Build history of the part. All positions in model axes, mm. A direction names the side the tool comes from. Round coordinates to 2 decimals unless told otherwise and drop trailing zeros. Order: outer loops, then holes, each group sorted by start corner. A loop starts at its lowest first (then second) coordinate and runs counter-clockwise, first axis right, second up. Notation, with made-up numbers: M 36.5,3 L 71.5,3 A14 ccw 71.5,7 Z; hole C -23.75,-25 d9. An arc over 180 degrees is marked long. Use CSV: the item, a comma, the result in double quotes.
from build123d import *

# Parameters (mm, degrees)
SKETCH1_R           = 2.95
SKETCH1_R_2         = 20
SKETCH1_R_3         = 18.5
BOSS_EXTRUDE1_DEPTH = 5.9
CUT_EXTRUDE2_DEPTH  = 78.081470808


with BuildPart() as part:
    # Sketch1 → Boss-Extrude1 (new body)
    with BuildSketch(Plane.XY):
        Polygon((-32.5, 4.1), (-32.5, -22), (32.5, -22), (32.5, 4.1), (54.344931419, 4.1), (54.344931419, 54.344931419), (-54.344931419, 54.344931419), (-54.344931419, 4.1), align=None)
        Circle(SKETCH1_R, mode=Mode.SUBTRACT)
        with Locations((29.344931419, 29.344931419)):
            Circle(SKETCH1_R_2, mode=Mode.SUBTRACT)
        with Locations((-29.344931419, 29.344931419)):
            Circle(SKETCH1_R_3, mode=Mode.SUBTRACT)
    extrude(amount=BOSS_EXTRUDE1_DEPTH)

    # Sketch3 → Cut-Extrude2 (cut, through all)
    with BuildSketch(Plane.XY.offset(5.9)):
        Polygon((-12.15, -22), (-7.85, -22), (-7.85, -17), (-5.4, -17), (-5.4, -14), (-7.85, -14), (-7.85, -10), (-12.15, -10), (-12.15, -14), (-14.6, -14), (-14.6, -17), (-12.15, -17), align=None)
        Polygon((7.85, -14), (7.85, -10), (12.15, -10), (12.15, -14), (14.6, -14), (14.6, -17), (12.15, -17), (12.15, -22), (7.85, -22), (7.85, -17), (5.4, -17), (5.4, -14), align=None)
    extrude(amount=-CUT_EXTRUDE2_DEPTH, mode=Mode.SUBTRACT)


solid = part.part
(1) Two-plate mould, pull along X, no slides. Class faces 1 (the face through (1, 54.345, 3)), 2 (the face through (-32.5, -9, 3)), 3 (the face through (32.5, -9, 3)), 4 (the face through (-14.6, -15, 3)): released by +X, released by -X, zero draft, split by the parting line, or undercut.
Answer block:
face 1,"zero draft"
face 2,"released by -X"
face 3,"released by +X"
face 4,"undercut"
(2) Cut at D-D, the plane y = 28. Give the cut face in (x, z).
Answer block:
outline,"M -54.34,0 L -47.8,0 L -47.8,5.9 L -54.34,5.9 Z; M -10.89,0 L 9.39,0 L 9.39,5.9 L -10.89,5.9 Z; M 49.3,0 L 54.34,0 L 54.34,5.9 L 49.3,5.9 Z"
(3) Wall check: line 1 (Y direction, x = 0, z = 3.55); line 2 (Y direction, x = 13, z = 5.2); line 3 (Y direction, x = -13, z = 1.35). Give the ranges that are in metal, low to high. Write a range as from..to.
Answer block:
line 1,"y = -22..-2.95, 2.95..54.34"
line 2,"y = -22..-17, -14..17.82, 40.87..54.34"
line 3,"y = -22..-17, -14..20.68, 38.01..54.34"
(4) Cut at C-C, the plane y = 12. Give the cut face in (x, z), and give its area (3 significant figures).
Answer block:
outline,"M -54.34,0 L -35.78,0 L -35.78,5.9 L -54.34,5.9 Z; M -22.91,0 L 19.39,0 L 19.39,5.9 L -22.91,5.9 Z; M 39.3,0 L 54.34,0 L 54.34,5.9 L 39.3,5.9 Z"
area,"448 mm²"
(5) Cut at B-B, the plane x = 0. Give the cut face in (y, z), and give its area (3 significant figures).
Answer block:
outline,"M -22,0 L -2.95,0 L -2.95,5.9 L -22,5.9 Z; M 2.95,0 L 54.34,0 L 54.34,5.9 L 2.95,5.9 Z"
area,"416 mm²"
(6) Tool access for faces 5 (the face through (-44, 4.1, 3)), 6 (the face through (-1, 17, 0)), 7 (the face through (-7, -14, 3)), 8 (the face through (22, -22, 3)), 9 (the face through (12.15, -19, 3)): list every direction of +Z, -Z, +X, -X, +Y, -Y with a clear straight run to the whole face (end or side of a thin tool).
Answer block:
face 5,"+Z, -Z, -X, -Y"
face 6,"-Z, +X, -X, +Y, -Y"
face 7,"+Z, -Z"
face 8,"+Z, -Z, +X, -X, -Y"
face 9,"+Z, -Z, -Y"
(7) Cut at A-A, the plane y = 0. Give the cut face in (x, z), and give its area (3 significant figures).
Answer block:
outline,"M -32.5,0 L -2.95,0 L -2.95,5.9 L -32.5,5.9 Z; M 2.95,0 L 32.5,0 L 32.5,5.9 L 2.95,5.9 Z"
area,"349 mm²"
(8) Drop flat-ended pins along their axis: pin 1 (2 mm diameter, centred on y = -9, z = 1.5, fed in from +X); pin 2 (1 mm diameter, centred on x = -36.5, z = 2, fed in from -Y); pin 3 (2.5 mm diameter, centred on y = -15.5, z = 2.5, fed in from -X). Give the stop position or say it passes through.
Answer block:
pin 1,"stops at x = 32.5"
pin 2,"stops at y = 4.1"
pin 3,"stops at x = -32.5"
